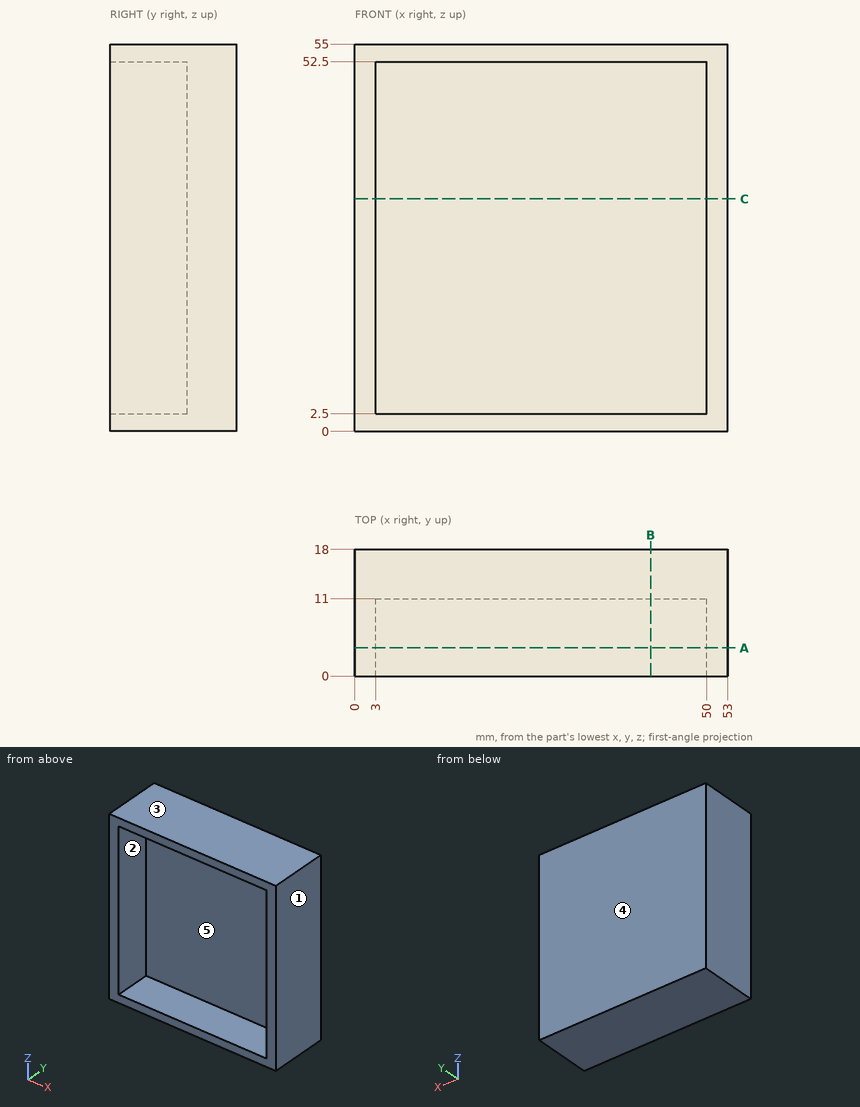
Print and shaded views of the part. All mm, measured from the part's lowest x, y and z. A direction names the side the tool comes from. Coordinates: 2 decimals unless noted, no trailing zeros. Order: outer loops, then holes, each group sorted by start corner. A loop starts at its lowest first (then second) coordinate and runs counter-clockwise, first axis right, second up. Notation, with made-up numbers: (-18, 85.5) - (9, 85.5) arc R34 cw to (9, 116.5) - close; hole circle Ø7 at (-7.75, 24.25). An arc over 180 degrees is marked (long way). Put each result on its own line as item: value.
1. Saw through at A-A (y = 4). Write the cut outline in (x, z), and give its area (3 significant figures).
Answer sheet:
outline: (0, 0) - (53, 0) - (53, 55) - (0, 55) - close; hole (3, 2.5) - (50, 2.5) - (50, 52.5) - (3, 52.5) - close
area: 565 mm^2
2. Pull direction Z, two halves, no side cores. Call the marked faces 1, 2 and 3: pulls with the +Z half, pulls with the -Z half, needs draft (parallel to the pull), parting line crosses it, or undercut.
Answer sheet:
face 1: needs draft
face 2: undercut
face 3: pulls with the +Z half
3. Saw through at B-B (x = 42). Write the cut outline in (y, z).
Answer sheet:
outline: (0, 0) - (18, 0) - (18, 55) - (0, 55) - (0, 52.5) - (11, 52.5) - (11, 2.5) - (0, 2.5) - close
4. Tool access for the marked faces 4 and 5: list every direction of +Z, -Z, +X, -X, +Y, -Y with a clear straight run to the whole face (end or side of a thin tool).
Answer sheet:
face 4: +Z, -Z, +X, -X, +Y
face 5: -Y
5. Probe line 1 along X through (y, z) = (2.5, 42); line 2 along Z through (x, y) = (29, 9.5); line 3 along Y through (x, z) = (28, 8). List the from-to ranges inside material, lowest first. Write a range as [from, to].
Answer sheet:
line 1: x = [0, 3], [50, 53]
line 2: z = [0, 2.5], [52.5, 55]
line 3: y = [11, 18]
6. Drop a flat-ended pin along its axis: P1, Ø23.5, axis at x = 21.5, z = 32, coming from the -Y side. Give the stop position or say it passes through.
Answer sheet:
P1: stops at y = 11
7. Saw through at C-C (z = 33). Write the cut outline in (x, y).
Answer sheet:
outline: (0, 0) - (3, 0) - (3, 11) - (50, 11) - (50, 0) - (53, 0) - (53, 18) - (0, 18) - close
